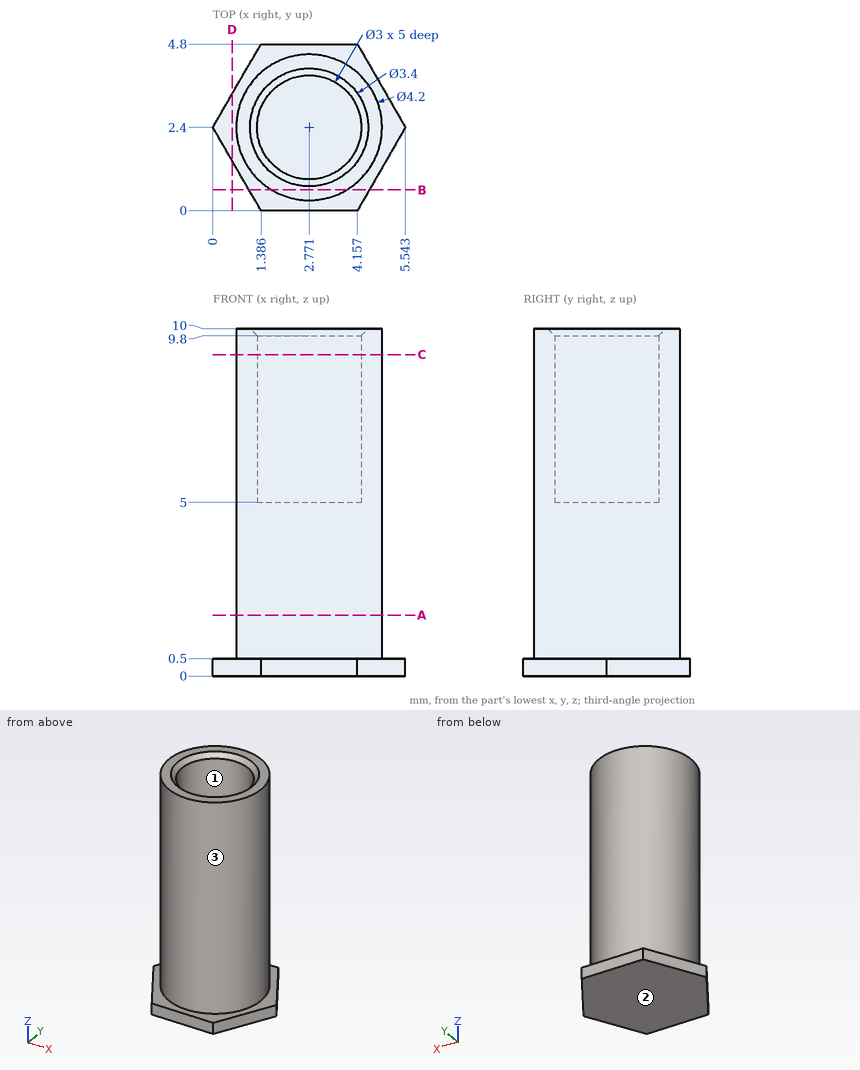
Part print with two shaded views. Sizes in mm from the minimum x, y, z corner. Give positions to 0.01 mm unless a question says otherwise; leave off trailing zeros. Order: outer loops, then holes, each group sorted by start corner. A loop starts at its lowest first (then second) coordinate and runs counter-clockwise, first axis right, second up.
1) Wall check: probe 1 along Y at (x, z) = (2.7, 7.5); probe 2 along Z at (x, y) = (1.5, 2); probe 3 along Z at (x, y) = (4.55, 3.85). Give the ranges that are in metal, low to high.
2) Saw through at A-A, the plane z = 1.75. Write the cut outline in (x, y).
3) Pin check, flat tips, straight feed: pin 1 (1.5 mm diameter, centred on y = 2, z = 5, fed in from +X); pin 2 (2.5 mm diameter, centred on x = 2.5, y = 1.5, fed in from +Z); pin 3 (1.5 mm diameter, centred on x = 4, z = 5, fed in from -Y) (1 decimal). Stop position of each tip, or through.
4) Mould opens along Y. For the marked faces 1, 2 and 3 say: +Y half, -Y half, draft (parallel to the pull), parting line (faces both ways), or undercut.
5) Saw through at D-D, the plane x = 0.55. Write the cut outline in (y, z).
6) Saw through at B-B, the plane y = 0.6. Write the cut outline in (x, z).
7) Saw through at C-C, the plane z = 9.25. Write the cut outline in (x, y).
Computed:
1. probe 1: y = 0.3 to 0.9, 3.9 to 4.5
1. probe 2: z = 0 to 5
1. probe 3: z = 0 to 0.5
2. outline: circle Ø4.2 at (2.77, 2.4)
3. pin 1: stops at x = 4.87
3. pin 2: stops at z = 10
3. pin 3: stops at y = 0.4
4. face 1: undercut
4. face 2: draft
4. face 3: parting line
5. outline: (1.45, 0) - (3.35, 0) - (3.35, 0.5) - (1.45, 0.5) - close
6. outline: (1.04, 0) - (4.5, 0) - (4.5, 0.5) - (3.85, 0.5) - (3.85, 10) - (1.69, 10) - (1.69, 0.5) - (1.04, 0.5) - close
7. outline: circle Ø4.2 at (2.77, 2.4); hole circle Ø3 at (2.77, 2.4)
